Verification items for the finished model (mm, model axes). A direction names the side the tool comes from. Round coordinates to 2 decimals unless told otherwise and drop trailing zeros. Write each loop counter-clockwise with the first axis right and the second up, starting at its lowest first coordinate (ties: lowest second). Pieces come first, ordered by that corner, then holes. Notation, with made-up numbers: M 36.25,50.25 L 77.25,50.25 A14 cw 77.25,59.25 Z; hole C -3,85.25 d3. An arc over 180 degrees is marked long. Answer in a Markdown table with one row per item. Add a question column.
1. Go/stop test with flat-tipped pins: pin 1 Ø5.5 at (y, z) = (3, 9.5) entering from +X; pin 2 Ø4 at (x, z) = (2.5, -2.5) entering from +Y; pin 3 Ø1.5 at (x, y) = (-10.5, -3) entering from -Z; pin 4 Ø1.5 at (x, y) = (0, 9.5) entering from +Z. Record where each tip stops, or that it passes through.
2. Material ranges on probe 1 along X at (y, z) = (8.75, 4); probe 2 along Y at (x, z) = (3.5, -8.25); probe 3 along X at (y, z) = (-3.75, 3.75), recorded low to high.
3. Sectioned sample at C-C on x = -9. Record the cut outline in (y, z).
4. Draft check along X on faces 1 (the flat face through (-6.25, 0, 10)), 2 (the flat face through (6.25, -10, 0)), 3 (the flat face through (-8, 0, -12.5)), 4 (the cylindrical face through (-11.359, 0.119, 11.297)). Enter one of: pulls with the +X half, pulls with the -X half, needs draft (parallel to the pull), parting line crosses it, or undercut.
5. Sectioned sample at A-A on y = -3.25. Record the cut outline in (x, z), plus the area to 3 significant figures.
6. Set-up check for faces 5 (the flat face through (-6.25, -10, 0)), 6 (the flat face through (10, 0, -6.25)), 7 (the flat face through (-6.25, 0, -10)): record each of +Z, -Z, +X, -X, +Y, -Y from which the full face is reachable in a straight line by a thin tool's end or side.
7. Sectioned sample at D-D on y = 9.5. Record the cut outline in (x, z), plus the area to 3 significant figures.
```python
from build123d import *

# Parameters (mm, degrees)
SKETCH1_W           = 25
SKETCH1_H           = 25
SKETCH1_W_2         = 12.5
SKETCH1_H_2         = 12.5
BOSS_EXTRUDE1_DEPTH = 12.5
SKETCH2_W           = 12.5
SKETCH2_H           = 12.5
CUT_EXTRUDE1_DEPTH  = 5
SKETCH3_W           = 12.5
SKETCH3_H           = 12.5
CUT_EXTRUDE2_DEPTH  = 5
SKETCH4_W           = 12.5
SKETCH4_H           = 12.5
CUT_EXTRUDE3_DEPTH  = 5
FILLET1_R           = 4


with BuildPart() as part:
    # Sketch1 → Boss-Extrude1 (new, symmetric)
    # profile 1 of 2: a face of its own
    with BuildSketch(Plane.XY):
        Rectangle(SKETCH1_W, SKETCH1_H)
        Rectangle(SKETCH1_W_2, SKETCH1_H_2, mode=Mode.SUBTRACT)
    # profile 2 of 2: a face of its own
    with BuildSketch(Plane.XY):
        Rectangle(SKETCH1_W_2, SKETCH1_H_2)
    extrude(amount=BOSS_EXTRUDE1_DEPTH, both=True)

    # Sketch2 → Cut-Extrude1 (cut)
    with BuildSketch(Plane(origin=(0, 0, -12.5), x_dir=(-1, 0, 0), z_dir=(0, 0, -1))):
        Rectangle(SKETCH2_W, SKETCH2_H)
    cut_extrude1 = extrude(amount=-CUT_EXTRUDE1_DEPTH, mode=Mode.SUBTRACT)

    # Mirror1: Cut-Extrude1 across plane
    add(cut_extrude1.mirror(Plane.XY), mode=Mode.SUBTRACT)

    # Sketch3 → Cut-Extrude2 (cut)
    with BuildSketch(Plane(origin=(0, 12.5, 0), x_dir=(1, 0, 0), z_dir=(0, 1, 0))):
        Rectangle(SKETCH3_W, SKETCH3_H)
    cut_extrude2 = extrude(amount=-CUT_EXTRUDE2_DEPTH, mode=Mode.SUBTRACT)

    # Sketch4 → Cut-Extrude3 (cut)
    with BuildSketch(Plane(origin=(12.5, 0, 0), x_dir=(0, 0, -1), z_dir=(1, 0, 0))):
        Rectangle(SKETCH4_W, SKETCH4_H)
    cut_extrude3 = extrude(amount=-CUT_EXTRUDE3_DEPTH, mode=Mode.SUBTRACT)

    # Mirror2: Cut-Extrude3 across plane
    add(cut_extrude3.mirror(Plane(origin=(0, 0, 0), x_dir=(0, 0, 1), z_dir=(1, 0, 0))), mode=Mode.SUBTRACT)

    # Mirror3: Cut-Extrude2 across plane
    add(cut_extrude2.mirror(Plane.ZX), mode=Mode.SUBTRACT)

    # Fillet1
    fillet1_edges = [part.edges().sort_by_distance(p)[0] for p in [
        (0, 12.5, 12.5),
        (-12.5, 0, 12.5),
        (0, -12.5, 12.5),
        (12.5, 0, 12.5),
        (0, -12.5, -12.5),
        (-12.5, 0, -12.5),
        (0, 12.5, -12.5),
        (12.5, 0, -12.5),
        (12.5, -12.5, 0),
        (-12.5, -12.5, 0),
        (-12.5, 12.5, 0),
        (12.5, 12.5, 0),
    ]]
    fillet(fillet1_edges, radius=FILLET1_R)


solid = part.part
```
Geometry check:
| question | item | result |
|---|---|---|
| 1 | pin 1 | stops at x = 12.5 |
| 1 | pin 2 | stops at y = 7.5 |
| 1 | pin 3 | stops at z = -12.3 |
| 1 | pin 4 | stops at z = 12.49 |
| 2 | probe 1 | x = -12.49 to -6.25, 6.25 to 12.49 |
| 2 | probe 2 | y = -12.5 to -6.25, 6.25 to 12.5 |
| 2 | probe 3 | x = -7.5 to 7.5 |
| 3 | outline | M -12.47,-8.5 A3.97 ccw -8.5,-12.47 L 8.5,-12.47 A3.97 ccw 12.47,-8.5 L 12.47,8.5 A3.97 ccw 8.5,12.47 L -8.5,12.47 A3.97 ccw -12.47,8.5 Z; hole M -6.25,-6.25 L 6.25,-6.25 L 6.25,6.25 L -6.25,6.25 Z |
| 4 | face 1 | undercut |
| 4 | face 2 | undercut |
| 4 | face 3 | needs draft |
| 4 | face 4 | pulls with the -X half |
| 5 | outline | M -12.5,-8.5 A4 ccw -8.5,-12.5 L -6.25,-12.5 L -6.25,-7.5 L 6.25,-7.5 L 6.25,-12.5 L 8.5,-12.5 A4 ccw 12.5,-8.5 L 12.5,-6.25 L 7.5,-6.25 L 7.5,6.25 L 12.5,6.25 L 12.5,8.5 A4 ccw 8.5,12.5 L 6.25,12.5 L 6.25,7.5 L -6.25,7.5 L -6.25,12.5 L -8.5,12.5 A4 ccw -12.5,8.5 L -12.5,6.25 L -7.5,6.25 L -7.5,-6.25 L -12.5,-6.25 Z |
| 5 | area | 361 mm2 |
| 6 | face 5 | -Y |
| 6 | face 6 | +X |
| 6 | face 7 | -Z |
| 7 | outline | M -12.37,-8.5 A3.87 ccw -8.5,-12.37 L 8.5,-12.37 A3.87 ccw 12.37,-8.5 L 12.37,8.5 A3.87 ccw 8.5,12.37 L -8.5,12.37 A3.87 ccw -12.37,8.5 Z; hole M -6.25,-6.25 L 6.25,-6.25 L 6.25,6.25 L -6.25,6.25 Z |
| 7 | area | 443 mm2 |
